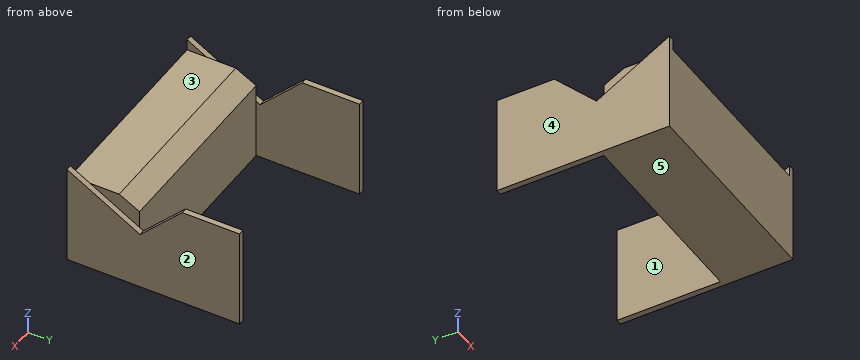
```python
from build123d import *

# Parameters (mm, degrees)
EXTRUDE_1_DEPTH     = 50
EXTRUDE_2_DEPTH     = 1720
EXTRUDE_START       = 1770
EXTRUDE_3_DEPTH     = 50
SKETCH_3_W          = 1820
SKETCH_3_H          = 1497
CUT_EXTRUDE_1_DEPTH = 850


with BuildPart() as part:
    # 草图1 → 凸台-拉伸1 (new body)
    with BuildSketch(Plane(origin=(0, 0, 0), x_dir=(0, 0, -1), z_dir=(1, 0, 0))):
        Polygon((0, 0), (365.848742481, 633.668609863), (0, 999.517352344), (0, 1497), (1722, 1497), (1722, 0), align=None)
    extrude(amount=EXTRUDE_1_DEPTH)

    # 草图2 → 凸台-拉伸2 (add)
    with BuildSketch(Plane(origin=(50, 0, 0), x_dir=(0, 0, -1), z_dir=(1, 0, 0))):
        Polygon((1722, 600), (194.068411452, 600), (98.124217521, 423), (98.124217521, 0), (1722, 0), align=None)
    extrude(amount=EXTRUDE_2_DEPTH)

    # 草图1<2> → 凸台-拉伸3 (add)
    with BuildSketch(Plane(origin=(0, 0, 0), x_dir=(0, 0, -1), z_dir=(1, 0, 0)).offset(EXTRUDE_START)):
        Polygon((0, 0), (365.848742481, 633.668609863), (0, 999.517352344), (0, 1497), (1722, 1497), (1722, 0), align=None)
    extrude(amount=EXTRUDE_3_DEPTH)

    # 草图3 → 切除-拉伸1 (cut)
    with BuildSketch(Plane(origin=(0, 0, -1722), x_dir=(-1, 0, 0), z_dir=(0, 0, -1))):
        with Locations((-910, 748.5)):
            Rectangle(SKETCH_3_W, SKETCH_3_H)
    extrude(amount=-CUT_EXTRUDE_1_DEPTH, mode=Mode.SUBTRACT)


solid = part.part
```
The model under review builds one solid part; all positions refer to its coordinate system, in mm. Face numbers are marked on the shaded views. A direction names the side the tool comes from. Round coordinates to 2 decimals unless told otherwise and drop trailing zeros. Write each loop counter-clockwise with the first axis right and the second up, starting at its lowest first coordinate (ties: lowest second). Pieces come first, ordered by that corner, then holes. Notation, with made-up numbers: (8, 56) - (19, 56) arc R18 ccw to (19, 74) - close; hole circle Ø3 at (32.25, 4). An arc over 180 degrees is marked (long way). Answer as CSV lines item,"result". Start each with the question number.
(1) We need section C-C on z = -762. State the section outline as (x, y) points.
(2) Draft analysis for pull direction X (two halves, no side actions). For the marked faces 3, 4 and 5, state which applies: pulls with the +X half, pulls with the -X half, needs draft (parallel to the pull), parting line crosses it, or undercut.
(3) We need section B-B on z = -223. State the section outline as (x, y) points, plus the area to 3 significant figures.
(4) For pin 1 Ø3 at (x, z) = (271.5, -737) entering from -Y, flat-tipped, find the tip position at first contact; note if it passes through.
(5) To check wall thickness, follow line 1 (X direction, y = 825, z = -274.5); line 2 (Y direction, x = 1024, z = -579); line 3 (Z direction, x = 439, y = 358). State the ranges of each line that lie inside material, in increasing order.
(6) We need section A-A on y = 1329.5. State the section outline as (x, z) points, plus the area to 3 significant figures.
(7) For the marked faces 1 and 2, list the 3-axis set-ups (+Z, -Z, +X, -X, +Y, -Y) from which the entire face can be reached by the end or side of a thin tool; tool diameter is ignored.
(8) We need section D-D on y = 503. State the section outline as (x, z) points.
Worked answers:
1,outline,"(0, 0) - (1820, 0) - (1820, 1497) - (1770, 1497) - (1770, 600) - (50, 600) - (50, 1497) - (0, 1497) - close"
2,face 3,"undercut"
2,face 4,"pulls with the -X half"
2,face 5,"needs draft"
3,outline,"(0, 0) - (1820, 0) - (1820, 386.25) - (1770, 386.25) - (1770, 600) - (50, 600) - (50, 386.25) - (0, 386.25) - close; (0, 776.52) - (50, 776.52) - (50, 1497) - (0, 1497) - close; (1770, 776.52) - (1820, 776.52) - (1820, 1497) - (1770, 1497) - close"
3,area,"1,140,000 mm²"
4,pin 1,"y = 0"
5,line 1,"0 to 50, 1770 to 1820"
5,line 2,"0 to 600"
5,line 3,"-872 to -98.12"
6,outline,"(0, -872) - (50, -872) - (50, 0) - (0, 0) - close; (1770, -872) - (1820, -872) - (1820, 0) - (1770, 0) - close"
6,area,"87,200 mm²"
7,face 1,"+Z, -Z, +Y"
7,face 2,"+Z, -Z, +X, +Y, -Y"
8,outline,"(0, -872) - (1820, -872) - (1820, -290.41) - (1770, -290.41) - (1770, -141.49) - (50, -141.49) - (50, -290.41) - (0, -290.41) - close"
